Build history of the part. All positions in model axes, mm. A direction names the side the tool comes from. Round coordinates to 2 decimals unless told otherwise and drop trailing zeros. Loops run counter-clockwise (first coordinate to the right, second up) from the corner with the lowest first, then second, coordinate; pieces in that order, holes last. Notation, with made-up numbers: M -28,22 L 27,22 A21 cw 27,48 Z; hole C -24,16.5 d5. An arc over 180 degrees is marked long. Use one line per item in the form item = value. Start each with the question number.
Autodesk Inventor part; units mm, degrees
ref_plane "YZ Plane" through (0, 0, 0) normal (1, 0, 0) x (0, 1, 0)
ref_plane "XZ Plane" through (0, 0, 0) normal (0, 1, 0) x (-1, 0, 0)
ref_plane "XY Plane" through (0, 0, 0) normal (0, 0, 1) x (1, 0, 0)
sketch "Sketch1" plane through (0, 0, 0) normal (0, 0, 1) x (1, 0, 0)
  line L0 (0, 0) -> (-179.3598, 0)
  line L1 (-179.3598, 0) -> (-179.3598, -1489.5)
  line L2 (-179.3598, -1489.5) -> (0, -1489.5)
  line L3 (0, -1489.5) -> (0, 0)
  line L4 (-179.3598, -1389.5) -> (-66, -1389.5)
  line L5 (-66, -1389.5) -> (-66, -1384.5)
  line L6 (-66, -1384.5) -> (-179.3598, -1384.5)
  line L7 (-179.3598, -1384.5) -> (-179.3598, -1389.5)
  line L8 (-179.3598, -892.8333) -> (-66, -892.8333)
  line L9 (-66, -892.8333) -> (-66, -887.8333)
  line L10 (-66, -887.8333) -> (-179.3598, -887.8333)
  line L11 (-179.3598, -887.8333) -> (-179.3598, -892.8333)
  line L12 (-179.3598, -396.1667) -> (-66, -396.1667)
  line L13 (-66, -396.1667) -> (-66, -391.1667)
  line L14 (-66, -391.1667) -> (-179.3598, -391.1667)
  line L15 (-179.3598, -391.1667) -> (-179.3598, -396.1667)
  circle A0 centre (-179.3598, -154.5) radius 30
  point P0 (-179.3598, -396.1667)
  point P1 (-179.3598, -124.5)
  point P2 (-179.3598, -184.5)
  dimension "d0" = 1489.5
  dimension "d1" = 179.3598
  dimension "d2" = 5
  dimension "d4" = 100
  dimension "d7" = 496.6667
  dimension "d23" = 66
  dimension "d28" = 60
  dimension "d30" = 1335
extrude "Plate1" add sketch "Sketch1" along normal blind 4 contours L3 L2 L1 L4 L5 L6 L8 L9 L10 L12 L13 L14 A0 L0
sketch "Sketch2" plane through (-4, 0, 0) normal (1, 0, 0) x (0, 1, 0)
  line L0 (-1489.5, 0) -> (0, 0)
  line L1 (0, 0) -> (0, 60)
  line L2 (0, 60) -> (-1489.5, 60)
  line L3 (-1489.5, 60) -> (-1489.5, 0)
edge flange "Flange1" height 60 angle 90 thickness 4 bend radius 4 thickness toward (1, 0, 0) relief tear relief width 4 relief depth 2 edges at (0, -744.75, 4) wall of the first edge with corners at (-4, -1489.5, 0) (-4, 0, 0) (-4, 0, 60) (-4, -1489.5, 60)
bend "Bend1"
corner "Corner1"
chamfer "Corner Chamfer1" distance 3 angle 45 6 edges at (-179.3598, -1389.5, 2) (-179.3598, -1384.5, 2) (-179.3598, -892.8333, 2) (-179.3598, -887.8333, 2) (-179.3598, -391.1667, 2) (-179.3598, -396.1667, 2)
equation "\"d0\" = Стрингер_длина"
equation "\"d1\" = стрингер_глубина_2"
equation "\"d2\" = паз_под_стрингер_толщина"
equation "\"d7\" = Шаг_шпангоутов"
equation "\"d23\" = паз_под_стрингер_глубина - Thickness"
equation "\"d28\" = 2 * радиус_выреза_под_сварку"
equation "\"d12\" = Thickness"
equation "\"d13\" = BendReliefWidth"
equation "\"d14\" = BendReliefDepth"
equation "\"d15\" = MinimumRemnant"
equation "\"d16\" = TransitionRadius"
equation "\"d17\" = ребро_усилителей"
equation "\"d19\" = BendRadius"
equation "\"d20\" = CornerReliefSize"
equation "\"d21\" = GapSize"
equation "\"d22\" = JacobiRadiusSize"
equation "\"BendRadius\" = Thickness"
equation "\"BendReliefWidth\" = Thickness"
equation "\"BendReliefDepth\" = 0.5 * Thickness"
equation "\"CornerReliefSize\" = 4 * Thickness"
equation "\"MinimumRemnant\" = 2 * Thickness"
equation "\"TransitionRadius\" = BendRadius"
equation "\"JacobiRadiusSize\" = BendRadius"
equation "\"GapSize\" = Thickness"
properties part number "GBK 0103 stringer 2" material "Steel"
Q1. Saw through at B-B (y = -1264.5). Give the cut face in (x, z), and give its area (3 significant figures).
Q2. Saw through at D-D (y = -154.5). Give the cut face in (x, z).
Q3. Drop flat-ended pins along their axis: P1, Ø8, axis at y = -1115.5, z = 19.5, coming from the +X side; P2, Ø5, axis at x = -124, y = -486.5, coming from the +Z side; P3, Ø10, axis at y = -1231, z = 31, coming from the -X side; P4, Ø4.5, axis at y = -890, z = 1, coming from the -X side. Give the stop position or say it passes through.
Q4. Wall check: probe 1 along Z at (x, y) = (-111.5, -879); probe 2 along X at (y, z) = (-709, 40). Give the ranges that are in metal, low to high.
Q5. Saw through at A-A (x = -97). Give the cut face in (y, z), and give its area (3 significant figures).
Q6. Saw through at C-C (z = 43.5). Give the cut face in (x, y), and give its area (3 significant figures).
Q7. Pull direction Y, two halves, no side cores. Call faces 3 (the face through (0, -734, 34)), 4 (the face through (-63, 0, 3)), 5 (the face through (-149.367, -153.84, 1.972)), 6 (the face through (-63, -1489.5, 3)): pulls with the +Y half, pulls with the -Y half, needs draft (parallel to the pull), parting line crosses it, or undercut.
Q8. Tool access for faces 1 (the face through (-95, -734, 4)), 2 (the face through (-95, -734, 0)): list every direction of +Z, -Z, +X, -X, +Y, -Y with a clear straight run to the whole face (end or side of a thin tool).
Filled in:
q1.outline = M -179.36,0 L -8,0 A8 ccw 0,8 L 0,60 L -4,60 L -4,8 A4 cw -8,4 L -179.36,4 Z
q1.area = 931 mm²
q2.outline = M -149.36,0 L -8,0 A8 ccw 0,8 L 0,60 L -4,60 L -4,8 A4 cw -8,4 L -149.36,4 Z
q3.P1 = 0
q3.P2 = 4
q3.P3 = -4
q3.P4 = -176.44
q4.probe_1 = 0 to 4
q4.probe_2 = -4 to 0
q5.outline = M -1489.5,0 L -1389.5,0 L -1389.5,4 L -1489.5,4 Z; M -1384.5,0 L -892.83,0 L -892.83,4 L -1384.5,4 Z; M -887.83,0 L -396.17,0 L -396.17,4 L -887.83,4 Z; M -391.17,0 L 0,0 L 0,4 L -391.17,4 Z
q5.area = 5,900 mm²
q6.outline = M -4,-1489.5 L 0,-1489.5 L 0,0 L -4,0 Z
q6.area = 5,960 mm²
q7.face_3 = needs draft
q7.face_4 = pulls with the +Y half
q7.face_5 = undercut
q7.face_6 = pulls with the -Y half
q8.face_1 = +Z, -X, +Y, -Y
q8.face_2 = -Z, +X, -X, +Y, -Y
